```python
from build123d import *

# Parameters (mm, degrees)
F0_W      = 113.012448
F0_H      = 123.940129
F1_DEPTH  = 76.454
F3_DEPTH  = 101.092
F5_DEPTH  = 99.568
F7_DEPTH  = 103.378
F8_W      = 11.922672
F8_H      = 25.046903
F8_W_2    = 12.908016
F9_DEPTH  = 2.286
F10_R     = 0.621429
F11_DEPTH = 0.6858
F12_R     = 26.550664
F13_DEPTH = 1.27
F15_DEPTH = 1.778
F17_DEPTH = 2.794
F18_R     = 8.329505
F18_R_2   = 6.092118
F19_DEPTH = 3.302
F21_DEPTH = 3.556
F23_DEPTH = 3.048
F25_DEPTH = 2.8956
F26_R     = 1.618614
F26_R_2   = 1.245405
F27_DEPTH = 2.8956
F29_DEPTH = 2.6924
F30_R     = 98.414689
F30_R_2   = 31.825087
F31_DEPTH = 92.964


with BuildPart() as f1:
    # F0 (on Top) → F1 (new body)
    with BuildSketch(Plane.XY):
        with Locations((4.576676, -1.209681)):
            Rectangle(F0_W, F0_H)
    extrude(amount=F1_DEPTH)

    # F2 (on face) → F3 (cut)
    with BuildSketch(Plane.XY.offset(76.454)):
        Polygon((-51.929548, 60.760383), (-51.929548, 0), (-14.090432, 60.760383), align=None)
    extrude(amount=-F3_DEPTH, mode=Mode.SUBTRACT)

    # F4 (on face) → F5 (cut)
    with BuildSketch(Plane.XY.offset(76.454)):
        Polygon((13.499225, 60.760383), (61.0829, 0), (61.0829, 60.760383), align=None)
    extrude(amount=-F5_DEPTH, mode=Mode.SUBTRACT)

    # F6 (on face) → F7 (cut)
    with BuildSketch(Plane.XY.offset(76.454)):
        Polygon((-14.090432, 60.760383), (-51.929548, 0), (-0.295603, 60.760383), align=None)
        Polygon((13.499225, 60.760383), (-0.295603, 60.760383), (61.0829, 0), align=None)
    extrude(amount=-F7_DEPTH, mode=Mode.SUBTRACT)

    # F8 (on face) → F9 (cut)
    with BuildSketch(Plane.XY.offset(76.454)):
        with Locations((-5.961336, -50.656295)):
            Rectangle(F8_W, F8_H)
        with Locations((6.454008, -50.656295)):
            Rectangle(F8_W_2, F8_H)
    extrude(amount=-F9_DEPTH, mode=Mode.SUBTRACT)

    # F10 (on face) → F11 (join)
    with BuildSketch(Plane.XY.offset(74.168)):
        with Locations((-1.345813, -50.279461)):
            Circle(F10_R)
        with Locations((1.885621, -50.238032)):
            Circle(F10_R)
    extrude(amount=F11_DEPTH)

    # F12 (on face) → F13 (cut)
    with BuildSketch(Plane.XY.offset(76.454)):
        with Locations((1.504538, 13.202349)):
            Circle(F12_R)
    extrude(amount=-F13_DEPTH, mode=Mode.SUBTRACT)

    # F14 (on face) → F15 (join)
    with BuildSketch(Plane.XY.offset(75.184)):
        Polygon((12.751438, 36.157132), (-12.751438, 34.419841), (-23.998337, 11.465057), (-9.742361, -9.752435), (15.760514, -8.015144), (27.007414, 14.93964), align=None)
        Polygon((-6.828518, -5.384374), (-18.758564, 11.125626), (-10.425508, 29.712349), (9.837595, 31.789072), (21.767641, 15.279072), (13.434584, -3.307651), align=None, mode=Mode.SUBTRACT)
    extrude(amount=F15_DEPTH)

    # F16 (on face) → F17 (join)
    with BuildSketch(Plane.XY.offset(75.184)):
        Polygon((-16.9584, 12.139062), (-7.321048, -1.878684), (9.637352, -0.541365), (16.9584, 14.8137), (7.321048, 28.831446), (-9.637352, 27.494127), align=None)
        Polygon((7.031429, 3.249008), (-5.34145, 2.273298), (-12.372879, 12.500671), (-7.031429, 23.703754), (5.34145, 24.679464), (12.372879, 14.452091), align=None, mode=Mode.SUBTRACT)
    extrude(amount=F17_DEPTH)

    # F18 (on face) → F19 (join)
    with BuildSketch(Plane.XY.offset(75.184)):
        with Locations((0, 14.219483)):
            Circle(F18_R)
        with Locations((0, 14.219483)):
            Circle(F18_R_2, mode=Mode.SUBTRACT)
    extrude(amount=F19_DEPTH)

    # F20 (on face) → F21 (join)
    with BuildSketch(Plane.XY.offset(75.184)):
        Polygon((-2.917235, 18.868994), (-5.485212, 14.017839), (-2.567977, 9.368329), (2.917235, 9.569973), (5.485212, 14.421128), (2.567977, 19.070638), align=None)
        Polygon((-2.18643, 10.301922), (-4.485922, 14.154206), (-2.299493, 18.071767), (2.18643, 18.137044), (4.485922, 14.28476), (2.299493, 10.367199), align=None, mode=Mode.SUBTRACT)
    extrude(amount=-F21_DEPTH)

    # F22 (on face) → F23 (join)
    with BuildSketch(Plane.XY.offset(75.184)):
        Polygon((-1.87018, 19.37121), (-5.396616, 15.175724), (-3.526437, 10.023997), (1.87018, 9.067756), (5.396616, 13.263243), (3.526437, 18.41497), align=None)
        Polygon((-2.822472, 11.049773), (-4.156286, 15.078961), (-1.333814, 18.248671), (2.822472, 17.389194), (4.156286, 13.360006), (1.333814, 10.190296), align=None, mode=Mode.SUBTRACT)
    extrude(amount=F23_DEPTH)

    # F24 (on face) → F25 (join)
    with BuildSketch(Plane.XY.offset(75.184)):
        Polygon((-0.955476, 17.510887), (-2.977351, 15.240268), (-2.021875, 12.353964), (0.955476, 11.738278), (2.977351, 14.008897), (2.021875, 16.895202), align=None)
        Polygon((-1.423189, 12.827654), (-2.267781, 14.958636), (-0.844592, 16.755565), (1.423189, 16.421512), (2.267781, 14.290529), (0.844592, 12.4936), align=None, mode=Mode.SUBTRACT)
    extrude(amount=F25_DEPTH)

    # F26 (on face) → F27 (join)
    with BuildSketch(Plane.XY.offset(75.184)):
        with Locations((0.137317, 14.769351)):
            Circle(F26_R)
        with Locations((0.137317, 14.769351)):
            Circle(F26_R_2, mode=Mode.SUBTRACT)
    extrude(amount=F27_DEPTH)

    # F28 (on face) → F29 (join)
    with BuildSketch(Plane.XY.offset(75.184)):
        Polygon((-0.110171, 15.806148), (-0.871044, 15.152074), (-0.685036, 14.166102), (0.261845, 13.834204), (1.022717, 14.488278), (0.836709, 15.47425), align=None)
        Polygon((-0.488767, 14.24752), (-0.7024, 15.022809), (-0.137796, 15.595465), (0.64044, 15.392832), (0.854073, 14.617543), (0.28947, 14.044887), align=None, mode=Mode.SUBTRACT)
    extrude(amount=F29_DEPTH)

    # F30 (on face) → F31 (cut)
    with BuildSketch(Plane.XY.offset(76.454)):
        with Locations((1.504538, 13.202349)):
            Circle(F30_R)
        with Locations((1.504538, 13.202349)):
            Circle(F30_R_2, mode=Mode.SUBTRACT)
    extrude(amount=-F31_DEPTH, mode=Mode.SUBTRACT)

    # F32: F1 across plane


with BuildPart() as f1_1:
    add(f1.part)
    add(f1.part.mirror(Plane.XY))


solid = f1_1.part
```
Part model, mm, in its own coordinate system. A direction names the side the tool comes from. Coordinates: 2 decimals unless noted, no trailing zeros. Order: outer loops, then holes, each group sorted by start corner. A loop starts at its lowest first (then second) coordinate and runs counter-clockwise, first axis right, second up. Notation, with made-up numbers: (69.25, 1.25) - (122.25, 1.25) arc R12 cw to (122.25, 22.25) - close; hole circle Ø2 at (-9, -22). An arc over 180 degrees is marked (long way). Return JSON: item names as keys, results as strings. Group by question number.
Item 1: Which spindle directions (+Z, -Z, +X, -X, +Y, -Y) get a long thin tool onto all of the face, cutting with end or side? Do faces 3 (the face through (-18, 2, -75.184)), 4 (the face through (-0.21, 13.19, 76.61)). Say none if no direction does.
Item 2: Pin check, flat tips, straight feed: pin 1 (10 mm diameter, centred on x = 11, y = 0.5, fed in from +Z); pin 2 (2 mm diameter, centred on x = -22, z = 39, fed in from -Y); pin 3 (2 mm diameter, centred on y = 0, z = 28.5, fed in from +X). Stop position of each tip, or through.
Item 3: Drill centre lines: probe 1 along Z at (x, y) = (3, -13); probe 2 along Z at (x, y) = (12, 42); probe 3 along X at (y, z) = (13.5, 20.5). Where is each one in solid material? Low to high. Write a range as from..to.
Item 4: Cut at A-A (z = -11.5). List the corners of the cut face in (x, y).
Item 5: Pull direction Y, two halves, no side cores. Call faces 1 (the face through (2, 16, 78.08)), 2 (the face through (1, 8, 78.486)): pulls with the +Y half, pulls with the -Y half, needs draft (parallel to the pull), parting line crosses it, or undercut.
Check values:
{
 "1": {"face 3": "-Z", "face 4": "+Z"},
 "2": {"pin 1": "stops at z = 77.98", "pin 2": "stops at y = -9.3", "pin 3": "stops at x = 30.9"},
 "3": {"probe 1": "z = -75.18..75.18", "probe 2": "z = -76.45..76.45", "probe 3": "x = -30.32..33.33"},
 "4": {"outline": "circle Ø63.65 at (1.5, 13.2)"},
 "5": {"face 1": "undercut", "face 2": "needs draft"}
}
